Geometry check sheet. Reference: drawing and pictorial views, mm from the part's lowest x, y, z. Give positions to 0.01 mm unless a question says otherwise; leave off trailing zeros. Order: outer loops, then holes, each group sorted by start corner. A loop starts at its lowest first (then second) coordinate and runs counter-clockwise, first axis right, second up. Notation, with made-up numbers: (11, -4.75) - (37, -4.75) arc R9 cw to (37, 9.25) - close; hole circle Ø9 at (31, -11.5). An arc over 180 degrees is marked (long way). Answer as a JSON object with one key per item and string values.
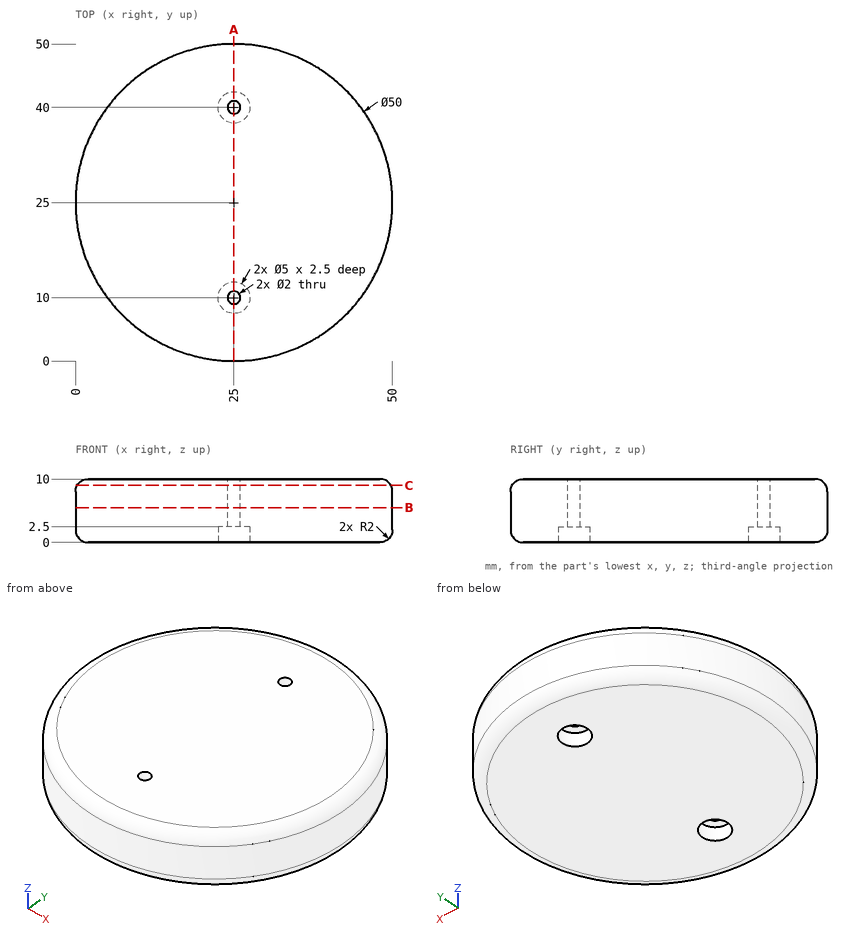
(1) Gauge pin test, flat ends, axial feed: pin 1 Ø1.5 at (y, z) = (8, 1) entering from -X; pin 2 Ø3 at (y, z) = (42.5, 7) entering from -X; pin 3 Ø2 at (x, z) = (25, 5.5) entering from -Y. Record the tip position at first contact, or that the pin passes through.
Computed values:
{"pin 1": "stops at x = 6.22", "pin 2": "stops at x = 5.79", "pin 3": "stops at y = 0"}
(2) Material ranges on line 1 along Y through (x, z) = (25, 4.25); line 2 along Y through (x, z) = (25, 1.85); line 3 along Z through (x, y) = (48.5, 28.5), recorded low to high. Write a range as [from, to].
Computed values:
{"line 1": "y = [0, 9], [11, 39], [41, 50]", "line 2": "y = [0.01, 7.5], [12.5, 37.5], [42.5, 49.99]", "line 3": "z = [0.15, 9.85]"}
(3) Section check B-B (z = 5.5). Record the cut outline in (x, y), then the cut area to 3 significant figures.
Computed values:
{"outline": "circle Ø50 at (25, 25); hole circle Ø2 at (25, 10); hole circle Ø2 at (25, 40)", "area": "1,960 mm²"}
(4) Section check A-A (x = 25). Record the cut outline in (y, z).
Computed values:
{"outline": "(0, 2) arc R2 ccw to (2, 0) - (7.5, 0) - (7.5, 2.5) - (9, 2.5) - (9, 10) - (2, 10) arc R2 ccw to (0, 8) - close; (11, 2.5) - (12.5, 2.5) - (12.5, 0) - (37.5, 0) - (37.5, 2.5) - (39, 2.5) - (39, 10) - (11, 10) - close; (41, 2.5) - (42.5, 2.5) - (42.5, 0) - (48, 0) arc R2 ccw to (50, 2) - (50, 8) arc R2 ccw to (48, 10) - (41, 10) - close"}
(5) Section check C-C (z = 9). Record the cut outline in (x, y).
Computed values:
{"outline": "circle Ø49.46 at (25, 25); hole circle Ø2 at (25, 10); hole circle Ø2 at (25, 40)"}
